The model under review builds one solid part; all positions refer to its coordinate system, in mm. A direction names the side the tool comes from. Round coordinates to 2 decimals unless told otherwise and drop trailing zeros. Order: outer loops, then holes, each group sorted by start corner. A loop starts at its lowest first (then second) coordinate and runs counter-clockwise, first axis right, second up. Notation, with made-up numbers: (81.25, -36) -> (89.25, -36) arc R23 cw to (89.25, 1) -> close; hole circle Ø3 at (-20.5, -1). An arc over 180 degrees is marked (long way). Return JSON: item names as keys, results as strings. Group by question number.
from build123d import *

# Parameters (mm, degrees)
F0_R     = 3
F0_R_2   = 2.25
F1_DEPTH = 10
F2_R     = 9.25
F2_R_2   = 3
F3_DEPTH = 3
F4_R     = 9.25
F4_R_2   = 8.5
F5_DEPTH = 10


with BuildPart() as f1:
    # F0 (on Front) → F1 (new body)
    with BuildSketch(Plane.XZ):
        Circle(F0_R)
        Circle(F0_R_2, mode=Mode.SUBTRACT)
    extrude(amount=F1_DEPTH)

    # F2 (on Front) → F3 (join)
    with BuildSketch(Plane.XZ):
        Circle(F2_R)
        Circle(F2_R_2, mode=Mode.SUBTRACT)
    extrude(amount=F3_DEPTH)

    # F4 (on face) → F5 (join)
    with BuildSketch(Plane(origin=(0, 0, 0), x_dir=(-1, 0, 0), z_dir=(0, 1, 0))):
        Circle(F4_R)
        Circle(F4_R_2, mode=Mode.SUBTRACT)
    extrude(amount=F5_DEPTH)


solid = f1.part
Item 1: The part is to be moulded in two halves that separate along X. For faces 1 (the face through (-3, -6, 0)), 2 (the face through (-4.57, 4.93, 7.167)), 3 (the face through (4, -3, 0)), say which applies: +X half, -X half, draft (parallel to the pull), parting line (faces both ways), or undercut.
Item 2: For faces 4 (the face through (2, 0, -2)), 5 (the face through (-0.29, -4.93, 2.23)), list the 3-axis set-ups (+Z, -Z, +X, -X, +Y, -Y) from which the entire face can be reached by the end or side of a thin tool; tool diameter is ignored.
Item 3: Consider section C-C on y = -7.5. State the section outline as (x, z) points.
Item 4: Consider section A-A on x = 0. State the section outline as (y, z) points, plus the area to 3 significant figures.
Item 5: Consider section D-D on z = -6. State the section outline as (x, y) points.
Item 6: Wall thickness on line 1 along Z through (x, y) = (0, -4); line 2 along Z through (x, y) = (0, 4.75); line 3 along Y through (x, z) = (7, -1.25): over which ranges is each line inside the solid? List them lowest first.
Item 7: Consider section B-B on z = 0. State the section outline as (x, y) points, plus the area to 3 significant figures.
Item 8: Insertion check: pin 1 Ø8 at (y, z) = (-5, 5.5) entering from -X; pin 2 Ø1.5 at (y, z) = (-0.5, -7) entering from +X; pin 3 Ø5 at (x, z) = (3, 3) entering from +Y. Each pin has a flat end and moves straight along its axis. Give the tip position at first contact, or say it passes through.
Values:
{
 "1": {"face 1": "parting line", "face 2": "undercut", "face 3": "draft"},
 "2": {"face 4": "+Y", "face 5": "+Y, -Y"},
 "3": {"outline": "circle Ø6 at (0, 0); hole circle Ø4.5 at (0, 0)"},
 "4": {"outline": "(-10, -3) -> (-3, -3) -> (-3, -9.25) -> (10, -9.25) -> (10, -8.5) -> (0, -8.5) -> (0, -2.25) -> (-10, -2.25) -> close; (-10, 2.25) -> (0, 2.25) -> (0, 8.5) -> (10, 8.5) -> (10, 9.25) -> (-3, 9.25) -> (-3, 3) -> (-10, 3) -> close", "area": "67.5 mm^2"},
 "5": {"outline": "(-7.04, -3) -> (7.04, -3) -> (7.04, 10) -> (6.02, 10) -> (6.02, 0) -> (-6.02, 0) -> (-6.02, 10) -> (-7.04, 10) -> close"},
 "6": {"line 1": "-3 to -2.25, 2.25 to 3", "line 2": "-9.25 to -8.5, 8.5 to 9.25", "line 3": "-3 to 0"},
 "7": {"outline": "(-9.25, -3) -> (-3, -3) -> (-3, -10) -> (-2.25, -10) -> (-2.25, 0) -> (-8.5, 0) -> (-8.5, 10) -> (-9.25, 10) -> close; (2.25, -10) -> (3, -10) -> (3, -3) -> (9.25, -3) -> (9.25, 10) -> (8.5, 10) -> (8.5, 0) -> (2.25, 0) -> close", "area": "67.5 mm^2"},
 "8": {"pin 1": "x = -9.02", "pin 2": "x = 6.82", "pin 3": "y = 0"}
}
